Verification items for this drawing (mm, ordinates from the low corner). A direction names the side the tool comes from. Give positions to 0.01 mm unless a question says otherwise; leave off trailing zeros. Order: outer loops, then holes, each group sorted by start corner. A loop starts at its lowest first (then second) coordinate and runs counter-clockwise, first axis right, second up. Notation, with made-up numbers: (10.5, 61.25) - (34.5, 61.25) arc R23 ccw to (34.5, 97.25) - close; hole circle Ø10 at (-38, 41). An arc over 180 degrees is marked (long way). Put each result on its own line as item: value. Start each with the question number.
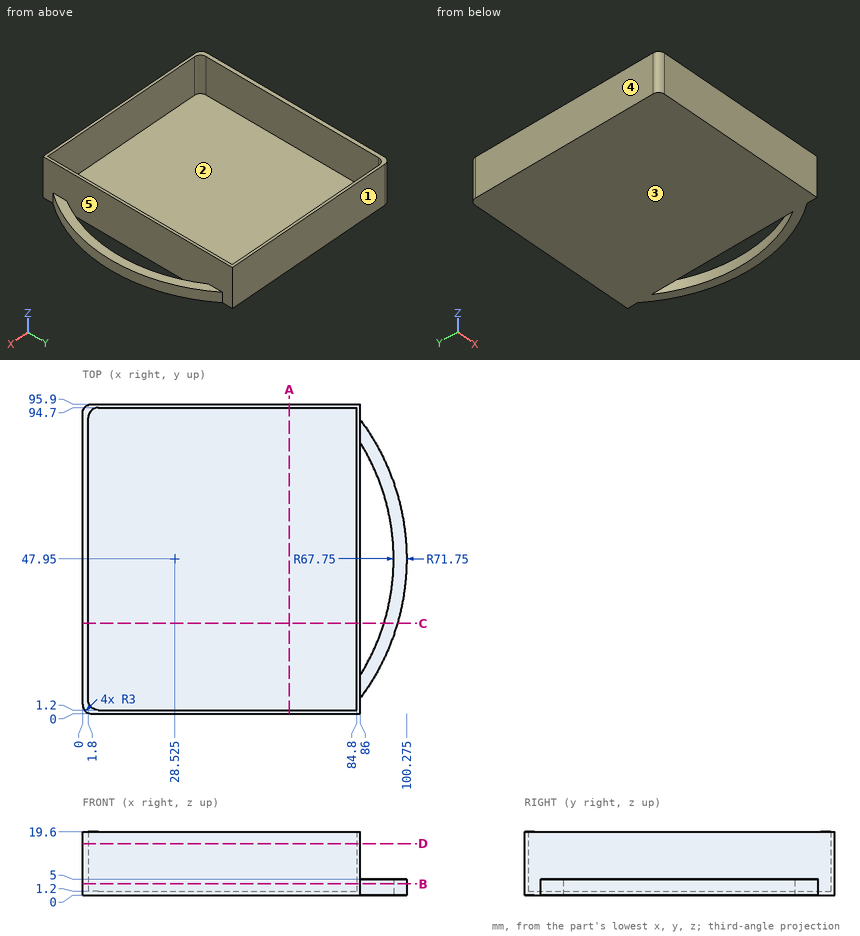
Item 1: Thickness scan on line 1 along Y through (x, z) = (10.5, 3); line 2 along X through (y, z) = (55.5, 6.5); line 3 along X through (y, z) = (24.5, 1.25) (1 decimal). Record the ranges inside material, lowest first.
Item 2: Set-up check for the marked faces 1 and 2: record each of +Z, -Z, +X, -X, +Y, -Y from which the full face is reachable in a straight line by a thin tool's end or side.
Item 3: Cross-section at B-B (z = 3.5). Count the separate pieces of the cut face and the enclosed holes in it, and give its area (3 significant figures).
Item 4: Cross-section at D-D (z = 16). Enter the section's corners in (x, y), and give its area (3 significant figures).
Item 5: Gauge pin test, flat ends, axial feed: pin 1 Ø7 at (x, y) = (92, 57.5) entering from +Z; pin 2 Ø1.5 at (x, y) = (22.5, 10) entering from +Z; pin 3 Ø3 at (y, z) = (70, 4) entering from +X. Record the tip position at first contact, or that the pin passes through.
Item 6: Cross-section at C-C (y = 28). Enter the section's corners in (x, z).
Item 7: Cross-section at A-A (x = 64). Enter the section's corners in (y, z).
Item 8: Release check for a two-part mould opening along X. For the marked faces 3, 4 and 5 record: +X half, -X half, draft (parallel to the pull), parting line (faces both ways), or undercut.
Recorded:
1. line 1: y = 0 to 1.2, 94.7 to 95.9
1. line 2: x = 0 to 1.8, 84.8 to 86
1. line 3: x = 0 to 1.8, 84.8 to 86, 92.1 to 96.3
2. face 1: +Z, -Z, +X, -X, +Y
2. face 2: +Z
3. separate pieces: 1
3. enclosed holes: 2
3. area: 823 mm^2
4. outline: (0, 3) arc R3 ccw to (3, 0) - (86, 0) - (86, 95.9) - (3, 95.9) arc R3 ccw to (0, 92.9) - close; hole (1.8, 4.2) arc R3 ccw to (4.8, 1.2) - (84.8, 1.2) - (84.8, 94.7) - (4.8, 94.7) arc R3 ccw to (1.8, 91.7) - close
4. area: 487 mm^2
5. pin 1: passes through
5. pin 2: stops at z = 1.2
5. pin 3: stops at x = 97.27
6. outline: (0, 0) - (86, 0) - (86, 19.6) - (84.8, 19.6) - (84.8, 1.2) - (1.8, 1.2) - (1.8, 19.6) - (0, 19.6) - close; (93.27, 0) - (97.45, 0) - (97.45, 5) - (93.27, 5) - close
7. outline: (0, 0) - (95.9, 0) - (95.9, 19.6) - (94.7, 19.6) - (94.7, 1.2) - (1.2, 1.2) - (1.2, 19.6) - (0, 19.6) - close
8. face 3: draft
8. face 4: -X half
8. face 5: undercut
